Could you check a few things on this model? Use its own coordinates, in mm. Coordinates: 2 decimals unless noted, no trailing zeros. Write each loop counter-clockwise with the first axis right and the second up, starting at its lowest first coordinate (ties: lowest second). Pieces come first, ordered by that corner, then holes. Notation, with made-up numbers: M 25.25,25.25 L 83.25,25.25 A33 cw 83.25,60.25 Z; hole C 57.25,27.5 d5. An arc over 180 degrees is marked long. Answer as CSV lines item,"result". Start each with the question number.
Item 1: Suppose I cut it at B-B, the plane x = 26. Write out the boundary of the cut face in (y, z).
Item 2: Suppose I cut it at C-C, the plane z = 1. Write out the boundary of the cut face in (x, y), and give its area (3 significant figures).
Item 3: I'm going to push a flat-ended pin straight in: P1, Ø3, axis at x = -25, y = 0, coming from the -Z side. Where does the tip first touch, or does it pass through?
Item 4: Suppose I cut it at A-A, the plane y = 0. Write out the boundary of the cut face in (x, z), and give its area (3 significant figures).
Item 5: Suppose I cut it at D-D, the plane y = -10.5. Write out the boundary of the cut face in (x, z).
Item 6: If I drill on line 1 along Y through (x, z) = (0, 0.65); line 2 along X through (y, z) = (-0.5, 2.35); line 3 along Y through (x, z) = (25, 0.65), over which ranges is the centre line in solid material (lowest first)? Write a range as [from, to].
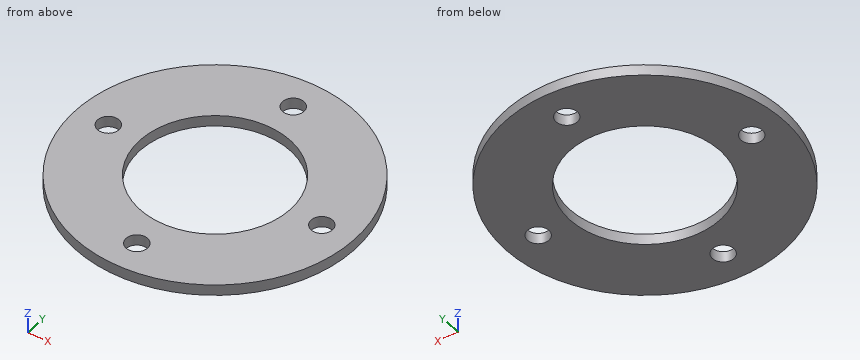
```python
from build123d import *

# Parameters (mm, degrees)
F0_R     = 32.5
F1_DEPTH = 2.54
F3_D     = 5
F4_R     = 17.5
F5_DEPTH = 2.541


with BuildPart() as f1:
    # F0 (on Top) → F1 (new body)
    with BuildSketch(Plane.XY):
        Circle(F0_R)
    extrude(amount=F1_DEPTH)

    # F3 (through all)
    with Locations(Plane.XY.offset(2.54)):
        with Locations((25, 0), (-25, 0), (0, -25), (0, 25)):
            Hole(F3_D / 2)

    # F4 (on face) → F5 (cut, through all)
    with BuildSketch(Plane.XY.offset(2.54)):
        Circle(F4_R)
    extrude(amount=-F5_DEPTH, mode=Mode.SUBTRACT)


solid = f1.part
```
Ans:
1,outline,"M -19.5,0 L -2.29,0 L -2.29,2.54 L -19.5,2.54 Z; M 2.29,0 L 19.5,0 L 19.5,2.54 L 2.29,2.54 Z"
2,outline,"C 0,0 d65; hole C -25,0 d5; hole C 0,0 d35; hole C 0,-25 d5; hole C 0,25 d5; hole C 25,0 d5"
2,area,"2,280 mm^2"
3,P1,"passes through"
4,outline,"M -32.5,0 L -27.5,0 L -27.5,2.54 L -32.5,2.54 Z; M -22.5,0 L -17.5,0 L -17.5,2.54 L -22.5,2.54 Z; M 17.5,0 L 22.5,0 L 22.5,2.54 L 17.5,2.54 Z; M 27.5,0 L 32.5,0 L 32.5,2.54 L 27.5,2.54 Z"
4,area,"50.8 mm^2"
5,outline,"M -30.76,0 L -14,0 L -14,2.54 L -30.76,2.54 Z; M 14,0 L 30.76,0 L 30.76,2.54 L 14,2.54 Z"
6,line 1,"y = [-32.5, -27.5], [-22.5, -17.5], [17.5, 22.5], [27.5, 32.5]"
6,line 2,"x = [-32.5, -27.45], [-22.55, -17.49], [17.49, 22.55], [27.45, 32.5]"
6,line 3,"y = [-20.77, -2.5], [2.5, 20.77]"
